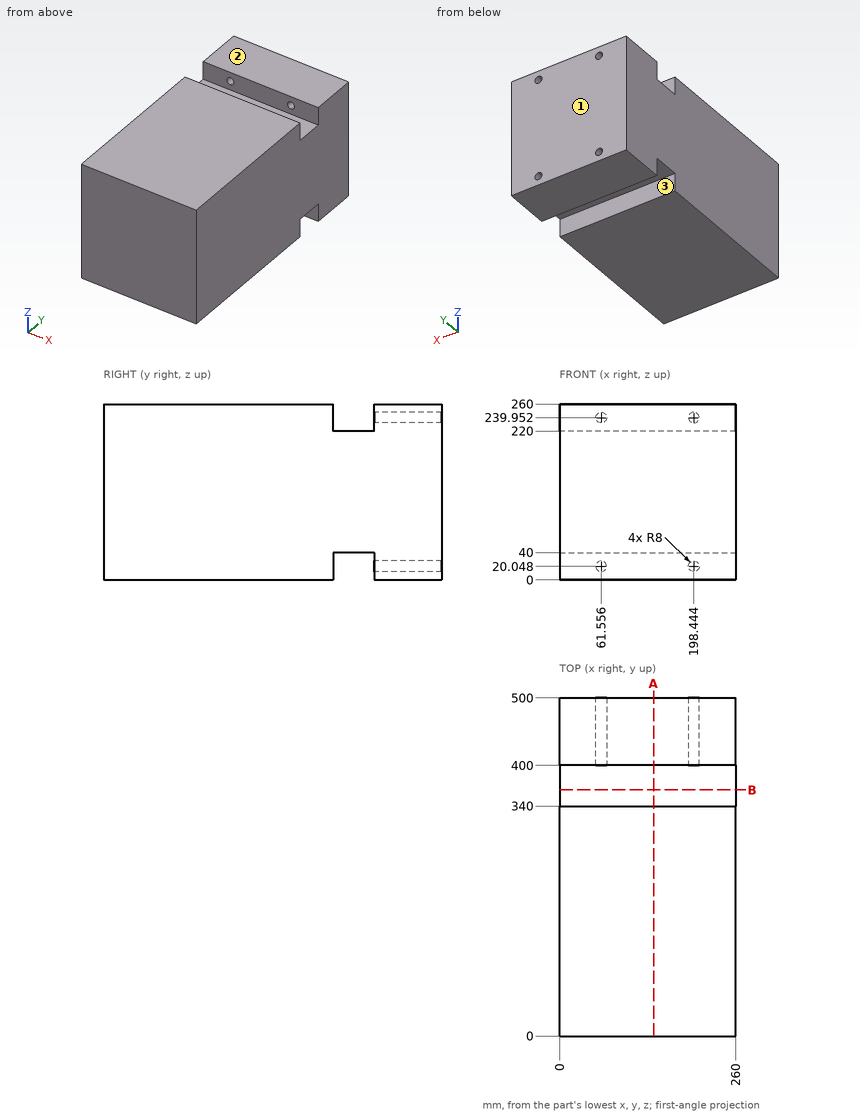
Check sheet for the drawn part. Datum: minimum x, y, z corner. Units: mm. Round coordinates to 2 decimals unless told otherwise and drop trailing zeros. Order: outer loops, then holes, each group sorted by start corner. A loop starts at its lowest first (then second) coordinate and runs counter-clockwise, first axis right, second up. Notation, with made-up numbers: M -27,-40 L 15,-40 A26 ccw 15,-18 Z; hole C 30,53.5 d3. An arc over 180 degrees is marked long. Answer in a Markdown table with one row per item.
(1) Gauge pin test, flat end, axial feed: pin 1 (5 mm diameter, centred on x = 158, z = 227, fed in from -Y). Record the tip position at first contact, or that the pin passes through.
Findings:
| item | result |
|---|---|
| pin 1 | stops at y = 0 |
(2) Material ranges on line 1 along Y through (x, z) = (199, 33); line 2 along Y through (x, z) = (196, 236); line 3 along Z through (x, y) = (239.5, 387.5), recorded low to high. Write a range as from..to.
Findings:
| item | result |
|---|---|
| line 1 | y = 0..340, 400..500 |
| line 2 | y = 0..340 |
| line 3 | z = 40..220 |
(3) Draft check along Y on the marked faces 1, 2 and 3. Enter one of: +Y half, -Y half, draft (parallel to the pull), parting line (faces both ways), or undercut.
Findings:
| item | result |
|---|---|
| face 1 | +Y half |
| face 2 | draft |
| face 3 | undercut |
(4) Section check B-B on y = 364. Record the boundary of the cut face in (x, z).
Findings:
| item | result |
|---|---|
| outline | M 0,40 L 260,40 L 260,220 L 0,220 Z |
(5) Section check A-A on x = 139. Record the boundary of the cut face in (y, z), plus the area to 3 significant figures.
Findings:
| item | result |
|---|---|
| outline | M 0,0 L 340,0 L 340,40 L 400,40 L 400,0 L 500,0 L 500,260 L 400,260 L 400,220 L 340,220 L 340,260 L 0,260 Z |
| area | 125,000 mm^2 |
